Here's how the part is built. I have some questions about the finished solid (model axes, mm). Face numbers are marked on the shaded views. A direction names the side the tool comes from. Coordinates: 2 decimals unless noted, no trailing zeros. Loops run counter-clockwise (first coordinate to the right, second up) from the corner with the lowest first, then second, coordinate; pieces in that order, holes last. Notation, with made-up numbers: (23.5, 66) - (67.5, 66) arc R21 ccw to (67.5, 92) - close; hole circle Ø7 at (79.5, 45.25). An arc over 180 degrees is marked (long way). Use a Markdown table: item, result.
```python
from build123d import *

# Parameters (mm, degrees)
BASE_EXTRUDE_DEPTH                           = 5
CUTAWAY_FOR_CLAMP_PLATE_WIRE_DEPTH           = 5
SKETCH3_R                                    = 2.413
CLAMP_PLATE_HOLES_ALTERED_TO_10_24_OCT_DEPTH = 5
HOLES_TO_PITCH_PLATE_REACH                   = 15.9
SKETCH4_R                                    = 2.286


with BuildPart() as part:
    # Sketch1 → Base-Extrude (new body, symmetric)
    with BuildSketch(Plane.XY):
        Polygon((-7.703086391, 2.967740731), (0, 0), (7.703086391, -2.967740731), (1.037503031, -20.268970563), (-27.810207986, -20.268970563), (-27.810207986, -6.368970563), (-11.300207986, -6.368970563), align=None)
    extrude(amount=BASE_EXTRUDE_DEPTH, both=True)

    # Sketch2 → Cutaway for Clamp Plate & Wire (cut)
    with BuildSketch(Plane.XY.offset(5)):
        Polygon((-7.703086391, 2.967740731), (7.703086391, -2.967740731), (1.037503031, -20.268970563), (-8.607332328, -20.268970563), (-4.290273371, -9.06358535), (-11.298169046, -6.363678277), align=None)
    extrude(amount=-CUTAWAY_FOR_CLAMP_PLATE_WIRE_DEPTH, mode=Mode.SUBTRACT)

    # Sketch3 → Clamp Plate Holes (altered to #10-24 OCT04) (cut)
    with BuildSketch(Plane.XY):
        with Locations((2.413510134, -5.216437969)):
            Circle(SKETCH3_R)
        with Locations((-5.289576257, -2.248697238)):
            Circle(SKETCH3_R)
    extrude(amount=-CLAMP_PLATE_HOLES_ALTERED_TO_10_24_OCT_DEPTH, mode=Mode.SUBTRACT)

    # Sketch4 → Holes to Pitch Plate (cut, up to next)
    with BuildSketch(Plane(origin=(0, -6.368970563, 0), x_dir=(-1, 0, 0), z_dir=(0, 1, 0)), mode=Mode.PRIVATE) as holes_to_pitch_plate_sk1:
        with Locations((23.682707986, 0)):
            Circle(SKETCH4_R)
    holes_to_pitch_plate_tool1 = extrude(holes_to_pitch_plate_sk1.sketch, amount=-HOLES_TO_PITCH_PLATE_REACH, mode=Mode.PRIVATE) & part.part
    add(holes_to_pitch_plate_tool1.solids().sort_by_distance((-23.682708, -6.368971, 0))[0], mode=Mode.SUBTRACT)
    # Sketch4 → Holes to Pitch Plate (cut, up to next)
    with BuildSketch(Plane(origin=(0, -6.368970563, 0), x_dir=(-1, 0, 0), z_dir=(0, 1, 0)), mode=Mode.PRIVATE) as holes_to_pitch_plate_sk2:
        with Locations(Location((15.427707986, 0, 0), (0, 0, 90))):  # turned: the seam where the file's is
            Circle(SKETCH4_R)
    holes_to_pitch_plate_tool2 = extrude(holes_to_pitch_plate_sk2.sketch, amount=-HOLES_TO_PITCH_PLATE_REACH, mode=Mode.PRIVATE) & part.part
    add(holes_to_pitch_plate_tool2.solids().sort_by_distance((-15.427708, -6.368971, 0))[0], mode=Mode.SUBTRACT)


solid = part.part
```
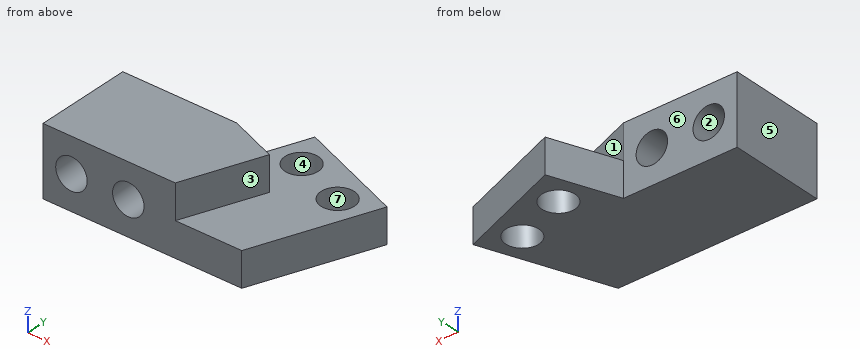
Q1. I want a section at B-B, the plane z = -1.25. Write out the boundary of the cut face in (x, y), then the cut area to 3 significant figures.
Check values:
| item | result |
|---|---|
| outline | (-27.81, -20.27) - (-25.6, -20.27) - (-25.6, -6.37) - (-27.81, -6.37) - close; (-21.77, -20.27) - (-17.34, -20.27) - (-17.34, -6.37) - (-21.77, -6.37) - close; (-13.51, -20.27) - (1.04, -20.27) - (7.7, -2.97) - (-7.7, 2.97) - (-11.3, -6.37) - (-13.51, -6.37) - close; hole circle Ø4.83 at (-5.29, -2.25); hole circle Ø4.83 at (2.41, -5.22) |
| area | 408 mm^2 |
Q2. Will these pins go through, and if not, where does the flat tip stop? P1, Ø2.5, axis at x = -23.68, z = 0, coming from the -Y side; P2, Ø7.5, axis at x = -5.29, y = -2.25, coming from the +Z side; P3, Ø5, axis at x = 1, z = -1, coming from the +Y side; P4, Ø2, axis at y = -4, z = -1, coming from the +X side.
Check values:
| item | result |
|---|---|
| P1 | through |
| P2 | z = 0 |
| P3 | y = 0.58 |
| P4 | x = 7.69 |
Q3. I want a section at C-C, the plane y = -7.25. Write out the boundary of the cut face in (x, z), then the cut area to 3 significant figures.
Check values:
| item | result |
|---|---|
| outline | (-27.81, -5) - (1.11, -5) - (1.11, 0) - (-9, 0) - (-9, 5) - (-27.81, 5) - close; (3.71, -5) - (6.05, -5) - (6.05, 0) - (3.71, 0) - close; hole circle Ø4.57 at (-23.68, 0); hole circle Ø4.57 at (-15.43, 0) |
| area | 218 mm^2 |
Q4. If we mould it in two halves opening along X, with no side actions, what happens to the marked faces 4, 5, 6 and 7? For each: pulls with the +X half, pulls with the -X half, needs draft (parallel to the pull), parting line crosses it, or undercut.
Check values:
| item | result |
|---|---|
| face 4 | undercut |
| face 5 | pulls with the -X half |
| face 6 | needs draft |
| face 7 | undercut |
Q5. I want a section at D-D, the plane z = 1. Give the number of separate pieces and of enclosed holes in the cut face, then the cut area to 3 significant figures.
Check values:
| item | result |
|---|---|
| separate pieces | 3 |
| enclosed holes | 0 |
| area | 179 mm^2 |
Q6. Which directions (+Z, -Z, +X, -X, +Y, -Y) give clear straight access to the entire face, cutting with the end or side of a thin tool? Please do the marked faces 1, 2 and 3.
Check values:
| item | result |
|---|---|
| face 1 | +Z, +X, +Y |
| face 2 | +Y, -Y |
| face 3 | +Z, +X, -Y |
Q7. Please list where these lines run through material, in increasing order: L1, parallel to Z at x = -23.5, y = -15.5; L2, parallel to X at y = -11, z = -0.5; L3, parallel to Z at x = -5.5, y = -13.25. Write a range as from..to.
Check values:
| item | result |
|---|---|
| L1 | -5..-2.28, 2.28..5 |
| L2 | -27.81..-25.91, -21.45..-17.66, -13.2..4.61 |
| L3 | -5..0 |
Q8. I want a section at A-A, the plane x = -14. Write out the boundary of the cut face in (y, z), then the cut area to 3 significant figures.
Check values:
| item | result |
|---|---|
| outline | (-20.27, -5) - (-6.37, -5) - (-6.37, -1.79) - (-20.27, -1.79) - close; (-20.27, 1.79) - (-6.37, 1.79) - (-6.37, 5) - (-20.27, 5) - close |
| area | 89.4 mm^2 |
